Geometry check sheet. Reference: drawing and pictorial views, mm from the part's lowest x, y, z. A direction names the side the tool comes from. Give positions to 0.01 mm unless a question says otherwise; leave off trailing zeros. Loops run counter-clockwise (first coordinate to the right, second up) from the corner with the lowest first, then second, coordinate; pieces in that order, holes last. Notation, with made-up numbers: M -4.5,44 L 51.5,44 A32 cw 51.5,82 Z; hole C 71.25,42.5 d6. An arc over 180 degrees is marked long. One line per question, with ' | ' between items. Start each with the question number.
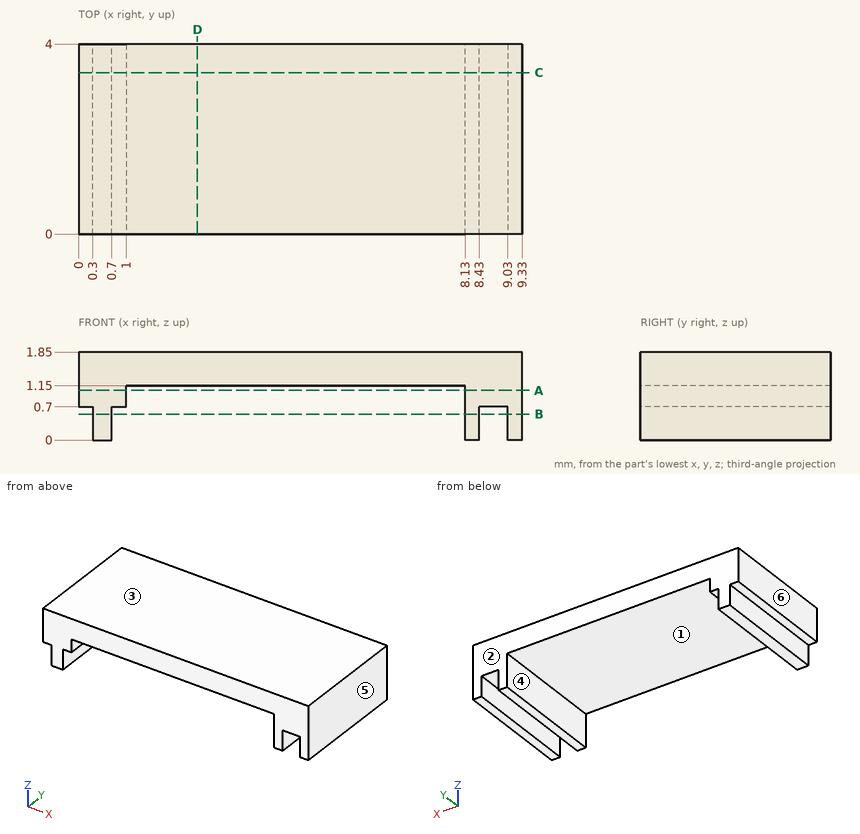
Q1. Cross-section at B-B (z = 0.55). Record the cut outline in (x, y).
Q2. Cross-section at D-D (x = 2.5). Record the cut outline in (y, z).
Q3. Cross-section at C-C (y = 3.4). Record the cut outline in (x, z).
Q4. Access from +Z, -Z, +X, -X, +Y, -Y to the whole of each face (thin tool, end or side, straight path). Record for the marked faces 1 and 2.
Q5. Draft check along X on the marked faces 3, 4, 5 and 6. Enter one of: released by +X, released by -X, zero draft, split by the parting line, or undercut.
Q6. Material ranges on probe 1 along X at (y, z) = (0.9, 0.25); probe 2 along X at (y, z) = (2.8, 0.8); probe 3 along Z at (x, y) = (4, 2.4), recorded low to high. Write a range as from..to.
Q7. Cross-section at A-A (z = 1.05). Record the cut outline in (x, y).
Solved:
1) outline: M 0.3,0 L 0.7,0 L 0.7,4 L 0.3,4 Z; M 8.13,0 L 8.43,0 L 8.43,4 L 8.13,4 Z; M 9.03,0 L 9.33,0 L 9.33,4 L 9.03,4 Z
2) outline: M 0,1.15 L 4,1.15 L 4,1.85 L 0,1.85 Z
3) outline: M 0,0.7 L 0.3,0.7 L 0.3,0 L 0.7,0 L 0.7,0.7 L 1,0.7 L 1,1.15 L 8.13,1.15 L 8.13,0 L 8.43,0 L 8.43,0.7 L 9.03,0.7 L 9.03,0 L 9.33,0 L 9.33,1.85 L 0,1.85 Z
4) face 1: -Z, +Y, -Y | face 2: +Z, -Z, +X, -X, +Y
5) face 3: zero draft | face 4: undercut | face 5: released by +X | face 6: released by -X
6) probe 1: x = 0.3..0.7, 8.13..8.43, 9.03..9.33 | probe 2: x = 0..1, 8.13..9.33 | probe 3: z = 1.15..1.85
7) outline: M 0,0 L 1,0 L 1,4 L 0,4 Z; M 8.13,0 L 9.33,0 L 9.33,4 L 8.13,4 Z
